from build123d import *

# Parameters (mm, degrees)
SKETCH_1_W          = 420
SKETCH_1_H          = 700
SKETCH_1_R          = 5
SKETCH_1_R_2        = 15
EXTRUDE_1_DEPTH     = 10
SKETCH_2_W          = 48.23
SKETCH_2_H          = 13.71
CUT_EXTRUDE_1_DEPTH = 10


with BuildPart() as part:
    # 草图1 → 凸台-拉伸1 (new body)
    with BuildSketch(Plane.XY):
        with Locations((210, 0)):
            Rectangle(SKETCH_1_W, SKETCH_1_H)
        with Locations((130, 114.5)):
            Circle(SKETCH_1_R, mode=Mode.SUBTRACT)
        with Locations((130, 15.5)):
            Circle(SKETCH_1_R, mode=Mode.SUBTRACT)
        with Locations((210, 114.5)):
            Circle(SKETCH_1_R, mode=Mode.SUBTRACT)
        with Locations((210, 15.5)):
            Circle(SKETCH_1_R, mode=Mode.SUBTRACT)
        with Locations((290, 114.5)):
            Circle(SKETCH_1_R, mode=Mode.SUBTRACT)
        with Locations((290, 15.5)):
            Circle(SKETCH_1_R, mode=Mode.SUBTRACT)
        with Locations((370, 114.5)):
            Circle(SKETCH_1_R, mode=Mode.SUBTRACT)
        with Locations((370, 15.5)):
            Circle(SKETCH_1_R, mode=Mode.SUBTRACT)
        with Locations((130, 65)):
            Circle(SKETCH_1_R_2, mode=Mode.SUBTRACT)
        with Locations((210, 65)):
            Circle(SKETCH_1_R_2, mode=Mode.SUBTRACT)
        with Locations((290, 65)):
            Circle(SKETCH_1_R_2, mode=Mode.SUBTRACT)
        with Locations((370, 65)):
            Circle(SKETCH_1_R_2, mode=Mode.SUBTRACT)
        with Locations((130, -114.5)):
            Circle(SKETCH_1_R, mode=Mode.SUBTRACT)
        with Locations((130, -15.5)):
            Circle(SKETCH_1_R, mode=Mode.SUBTRACT)
        with Locations((210, -114.5)):
            Circle(SKETCH_1_R, mode=Mode.SUBTRACT)
        with Locations((210, -15.5)):
            Circle(SKETCH_1_R, mode=Mode.SUBTRACT)
        with Locations((290, -114.5)):
            Circle(SKETCH_1_R, mode=Mode.SUBTRACT)
        with Locations((290, -15.5)):
            Circle(SKETCH_1_R, mode=Mode.SUBTRACT)
        with Locations((370, -114.5)):
            Circle(SKETCH_1_R, mode=Mode.SUBTRACT)
        with Locations((370, -15.5)):
            Circle(SKETCH_1_R, mode=Mode.SUBTRACT)
        with Locations((130, -65)):
            Circle(SKETCH_1_R_2, mode=Mode.SUBTRACT)
        with Locations((210, -65)):
            Circle(SKETCH_1_R_2, mode=Mode.SUBTRACT)
        with Locations((290, -65)):
            Circle(SKETCH_1_R_2, mode=Mode.SUBTRACT)
        with Locations((370, -65)):
            Circle(SKETCH_1_R_2, mode=Mode.SUBTRACT)
    extrude(amount=EXTRUDE_1_DEPTH)

    # 草图2 → 切除-拉伸1 (cut)
    with BuildSketch(Plane(origin=(0, 0, 0), x_dir=(-1, 0, 0), z_dir=(0, 0, -1))):
        with Locations((-33.645, 268.145)):
            Rectangle(SKETCH_2_W, SKETCH_2_H)
    extrude(amount=-CUT_EXTRUDE_1_DEPTH, mode=Mode.SUBTRACT)


solid = part.part
The model under review builds one solid part; all positions refer to its coordinate system, in mm. Round coordinates to 2 decimals unless told otherwise and drop trailing zeros. Write each loop counter-clockwise with the first axis right and the second up, starting at its lowest first coordinate (ties: lowest second). Pieces come first, ordered by that corner, then holes. Notation, with made-up numbers: M -5,83.5 L 42,83.5 A9 ccw 42,89.5 Z; hole C 36.5,-5 d4. An arc over 180 degrees is marked long. Use a Markdown table: item, result. Add a question column.
Q1. We need section A-A, the plane y = -65. State the section outline as (x, z) points.
Q2. We need section B-B, the plane z = 7. Count the separate pieces of the cut face and the enclosed holes in it, plus the area to 3 significant figures.
Q3. The part is to be moulded in two halves that separate along X. For faces 1 (the face through (206.748, 50.357, 4.93)), 2 (the face through (383.856, 59.255, 4.93)), 3 (the face through (207, 5, 10)), say which applies: pulls with the +X half, pulls with the -X half, needs draft (parallel to the pull), parting line crosses it, or undercut.
Q4. To check wall thickness, follow line 1 (Y direction, x = 296, z = 7.25); line 2 (X direction, y = -119, z = 2); line 3 (Y direction, x = 375.5, z = 9.5). State the ranges of each line that lie inside material, in increasing order.
Findings below:
| question | item | result |
|---|---|---|
| 1 | outline | M 0,0 L 115,0 L 115,10 L 0,10 Z; M 145,0 L 195,0 L 195,10 L 145,10 Z; M 225,0 L 275,0 L 275,10 L 225,10 Z; M 305,0 L 355,0 L 355,10 L 305,10 Z; M 385,0 L 420,0 L 420,10 L 385,10 Z |
| 2 | separate pieces | 1 |
| 2 | enclosed holes | 25 |
| 2 | area | 286,000 mm² |
| 3 | face 1 | undercut |
| 3 | face 2 | undercut |
| 3 | face 3 | needs draft |
| 4 | line 1 | y = -350 to -78.75, -51.25 to 51.25, 78.75 to 350 |
| 4 | line 2 | x = 0 to 127.82, 132.18 to 207.82, 212.18 to 287.82, 292.18 to 367.82, 372.18 to 420 |
| 4 | line 3 | y = -350 to -78.96, -51.04 to 51.04, 78.96 to 350 |
